Verification items for the finished model (mm, model axes). Round coordinates to 2 decimals unless told otherwise and drop trailing zeros. Loops run counter-clockwise (first coordinate to the right, second up) from the corner with the lowest first, then second, coordinate; pieces in that order, holes last. Notation, with made-up numbers: (13, 11.5) - (58, 11.5) arc R31 ccw to (58, 47.5) - close; hole circle Ø5 at (42.25, 6). An arc over 180 degrees is marked (long way). Use a Markdown table: item, result. Add a question column.
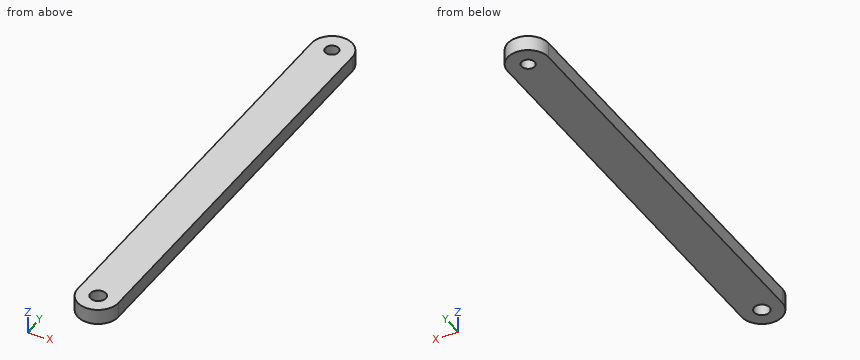
```python
from build123d import *

# Parameters (mm, degrees)
MODEL_R             = 1.5
MODEL_R_2           = 1.3
BOSS_EXTRUDE1_DEPTH = 3


with BuildPart() as part:
    # Model → Boss-Extrude1 (new body)
    with BuildSketch(Plane.XY):
        with BuildLine():
            Line((47.500099999, 80.00015), (47.500099999, 4.9999e-05))
            ThreePointArc((47.500099999, 4.9999e-05), (51.499999999, -3.99985), (55.499899998, 4.9999e-05))
            Line((55.499899998, 4.9999e-05), (55.483779921, 0))
            Line((55.483779921, 0), (55.499899998, 80.000050001))
            ThreePointArc((55.499899998, 80.000050001), (51.500049998, 84), (47.500099999, 80.00015))
        make_face()
        with Locations((51.500099998, 4.9998e-05)):
            Circle(MODEL_R, mode=Mode.SUBTRACT)
        with Locations((51.500099998, 80.000049998)):
            Circle(MODEL_R_2, mode=Mode.SUBTRACT)
    extrude(amount=BOSS_EXTRUDE1_DEPTH)


solid = part.part
```
Q1. Thickness scan on line 1 along Y through (x, z) = (52, 1.8); line 2 along X through (y, z) = (14.5, 0.9); line 3 along Y through (x, z) = (48.5, 0.2). Record the ranges inside material, lowest first.
Q2. Go/stop test with flat-tipped pins: pin 1 Ø1.5 at (y, z) = (22.5, 1) entering from +X; pin 2 Ø2.5 at (x, y) = (51.5, 0) entering from -Z. Record where each tip stops, or that it passes through.
Q3. Section check B-B on x = 51.5. Record the cut outline in (y, z).
Q4. Section check A-A on z = 2.55. State how many separate pieces and enclosed holes the cut face has, plus the area to 3 significant figures.
Determined:
| question | item | result |
|---|---|---|
| 1 | line 1 | y = -3.97 to -1.41, 1.41 to 78.8, 81.2 to 83.97 |
| 1 | line 2 | x = 47.5 to 55.49 |
| 1 | line 3 | y = -2.65 to 82.65 |
| 2 | pin 1 | stops at x = 55.49 |
| 2 | pin 2 | passes through |
| 3 | outline | (-4, 0) - (-1.5, 0) - (-1.5, 3) - (-4, 3) - close; (1.5, 0) - (78.7, 0) - (78.7, 3) - (1.5, 3) - close; (81.3, 0) - (84, 0) - (84, 3) - (81.3, 3) - close |
| 4 | separate pieces | 1 |
| 4 | enclosed holes | 2 |
| 4 | area | 677 mm² |
